CAD build for the part. Positions are in the model's coordinates, mm. Face numbers are marked on the shaded views. A direction names the side the tool comes from. Round coordinates to 2 decimals unless told otherwise and drop trailing zeros. Write each loop counter-clockwise with the first axis right and the second up, starting at its lowest first coordinate (ties: lowest second). Pieces come first, ordered by that corner, then holes. Notation, with made-up numbers: (73, -28) - (99, -28) arc R26 cw to (99, 3) - close; hole circle Ø9 at (80, 64.5). An arc over 180 degrees is marked (long way). Answer in a Markdown table with one row per item.
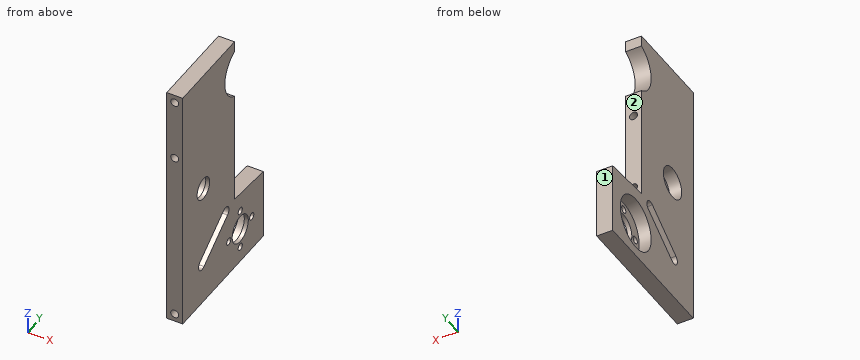
```python
from build123d import *

# Parameters (mm, degrees)
ESQUISSE2_W             = 8
ESQUISSE2_H             = 95
ESQUISSE2_H_2           = 31
BOSS_EXTRU_1_DEPTH      = 70
ESQUISSE3_R             = 7.95
ENL_V_MAT_EXTRU_1_DEPTH = 10
ESQUISSE4_R             = 13.4
ENL_V_MAT_EXTRU_2_DEPTH = 6
ESQUISSE6_R             = 1.8
ESQUISSE6_R_2           = 7
ENL_V_MAT_EXTRU_3_DEPTH = 10
ESQUISSE7_R             = 2
ENL_V_MAT_EXTRU_4_DEPTH = 15
ENL_V_MAT_EXTRU_5_DEPTH = 10
ESQUISSE9_R             = 13.4
ENL_V_MAT_EXTRU_6_DEPTH = 10
ESQUISSE10_R            = 13.4
ENL_V_MAT_EXTRU_7_DEPTH = 10
ESQUISSE12_R            = 8.1
ESQUISSE12_R_2          = 5.5
BOSS_EXTRU_3_DEPTH      = 2
ESQUISSE13_R            = 2
ENL_V_MAT_EXTRU_8_DEPTH = 15


with BuildPart() as part:
    # Esquisse2 → Boss.-Extru.1 (new body)
    with BuildSketch(Plane(origin=(0, 0, 0), x_dir=(1, 0, 0), z_dir=(0, 1, 0))):
        with Locations((4, 47.5)):
            Rectangle(ESQUISSE2_W, ESQUISSE2_H)
        with Locations((4, -15.5)):
            Rectangle(ESQUISSE2_W, ESQUISSE2_H_2)
    extrude(amount=BOSS_EXTRU_1_DEPTH)

    # Esquisse3 → Enlèv. mat.-Extru.1 (cut)
    with BuildSketch(Plane.ZY):
        with Locations((-32, 18)):
            Circle(ESQUISSE3_R)
    extrude(amount=-ENL_V_MAT_EXTRU_1_DEPTH, mode=Mode.SUBTRACT)

    # Esquisse4 → Enlèv. mat.-Extru.2 (cut)
    with BuildSketch(Plane.ZY):
        with Locations((-77, 50)):
            Circle(ESQUISSE4_R)
    extrude(amount=-ENL_V_MAT_EXTRU_2_DEPTH, mode=Mode.SUBTRACT)

    # Esquisse6 → Enlèv. mat.-Extru.3 (cut)
    with BuildSketch(Plane.ZY):
        with Locations((-77, 60)):
            Circle(ESQUISSE6_R)
        with Locations((-67, 50)):
            Circle(ESQUISSE6_R)
        with Locations((-77, 40)):
            Circle(ESQUISSE6_R)
        with Locations((-87, 50)):
            Circle(ESQUISSE6_R)
        with Locations((-77, 50)):
            Circle(ESQUISSE6_R_2)
    extrude(amount=-ENL_V_MAT_EXTRU_3_DEPTH, mode=Mode.SUBTRACT)

    # Esquisse7 → Enlèv. mat.-Extru.4 (cut)
    with BuildSketch(Plane.XZ):
        with Locations((4, -91)):
            Circle(ESQUISSE7_R)
        with Locations((4, -4)):
            Circle(ESQUISSE7_R)
        with Locations((4, 27)):
            Circle(ESQUISSE7_R)
    extrude(amount=-ENL_V_MAT_EXTRU_4_DEPTH, mode=Mode.SUBTRACT)

    # Esquisse8 → Enlèv. mat.-Extru.5 (cut)
    with BuildSketch(Plane.ZY):
        with BuildLine():
            Line((-61.528438992, 38.971206009), (-75.867849901, 18.492404902))
            ThreePointArc((-75.867849901, 18.492404902), (-75.131123077, 14.31421946), (-70.952937635, 15.050946284))
            Line((-70.952937635, 15.050946284), (-56.613526727, 35.529747391))
            ThreePointArc((-56.613526727, 35.529747391), (-57.35025355, 39.707932833), (-61.528438992, 38.971206009))
        make_face()
    extrude(amount=-ENL_V_MAT_EXTRU_5_DEPTH, mode=Mode.SUBTRACT)

    # Esquisse9 → Enlèv. mat.-Extru.6 (cut)
    with BuildSketch(Plane.ZY):
        with Locations((13, 50)):
            Circle(ESQUISSE9_R)
    extrude(amount=-ENL_V_MAT_EXTRU_6_DEPTH, mode=Mode.SUBTRACT)

    # Esquisse10 → Enlèv. mat.-Extru.7 (cut)
    with BuildSketch(Plane.ZY):
        with Locations((13, 50)):
            Circle(ESQUISSE10_R)
        Polygon((-57, 45), (-59, 70), (31, 70), (31, 45), align=None)
        with BuildLine():
            ThreePointArc((0.567783786, 45), (13, 36.6), (25.432216214, 45))
            Line((25.432216214, 45), (0.567783786, 45))
        make_face()
        with BuildLine():
            Line((0.567783786, 45), (25.432216214, 45))
            ThreePointArc((25.432216214, 45), (26.155829455, 47.453600313), (26.4, 50))
            ThreePointArc((26.4, 50), (10.453600313, 63.155829455), (0.567783786, 45))
        make_face()
    extrude(amount=-ENL_V_MAT_EXTRU_7_DEPTH, mode=Mode.SUBTRACT)

    # Esquisse12 → Boss.-Extru.3 (add)
    with BuildSketch(Plane(origin=(8, 0, 0), x_dir=(0, 0, -1), z_dir=(1, 0, 0))):
        with Locations((32, 18)):
            Circle(ESQUISSE12_R)
        with Locations((32, 18)):
            Circle(ESQUISSE12_R_2, mode=Mode.SUBTRACT)
    extrude(amount=-BOSS_EXTRU_3_DEPTH)

    # Esquisse13 → Enlèv. mat.-Extru.8 (cut)
    with BuildSketch(Plane(origin=(0, 45, 0), x_dir=(1, 0, 0), z_dir=(0, 1, 0))):
        with Locations((4, 12)):
            Circle(ESQUISSE13_R)
        with Locations((4, 52)):
            Circle(ESQUISSE13_R)
    extrude(amount=-ENL_V_MAT_EXTRU_8_DEPTH, mode=Mode.SUBTRACT)


solid = part.part
```
Q1. Drill centre lines: line 1 (Y direction, x = 6.65, z = -77); line 2 (Z direction, x = 4, y = 4); line 3 (Y direction, x = 4.25, z = -68.5). Where is each one in solid material? Low to high.
Computed:
| item | result |
|---|---|
| line 1 | y = 0 to 38.2, 41.8 to 43, 57 to 58.2, 61.8 to 70 |
| line 2 | z = -95 to -93, -89 to -6, -2 to 25, 29 to 31 |
| line 3 | y = 0 to 18.55, 29.01 to 39.64, 60.36 to 70 |
Q2. Saw through at C-C on y = 6. List the corners of the cut face in (x, z).
Computed:
| item | result |
|---|---|
| outline | (0, -95) - (8, -95) - (8, 31) - (0, 31) - close; hole circle Ø4 at (4, -91); hole circle Ø4 at (4, -4); hole circle Ø4 at (4, 27) |
Q3. Saw through at B-B on y = 31.5. List the corners of the cut face in (x, z), then the cut area to 3 significant figures.
Computed:
| item | result |
|---|---|
| outline | (0, -95) - (8, -95) - (8, -66.76) - (0, -66.76) - close; (0, -59.44) - (8, -59.44) - (8, 31) - (0, 31) - close; hole circle Ø4 at (4, -52); hole circle Ø4 at (4, -12) |
| area | 924 mm2 |
Q4. 3-axis set-ups, long thin cutter, end or side, ignore diameter. For the marked faces 1 and 2: which of +Z, -Z, +X, -X, +Y, -Y reach the whole face in a straight line?
Computed:
| item | result |
|---|---|
| face 1 | +Z, -Z, +X, -X, +Y |
| face 2 | +Z, +X, -X, +Y |
Q5. Saw through at A-A on x = 4. Count the separate pieces of the cut face and the enclosed holes in it, then the cut area to 3 significant figures.
Computed:
| item | result |
|---|---|
| separate pieces | 1 |
| enclosed holes | 3 |
| area | 5,200 mm2 |
Q6. Flat gauge pins, fed straight in: pin 1 (4 mm diameter, centred on x = 4.5, z = -27, fed in from +Y); pin 2 (4 mm diameter, centred on y = 50, z = -87, fed in from -X). Where does each tip first touch, or does it go through?
Computed:
| item | result |
|---|---|
| pin 1 | stops at y = 45 |
| pin 2 | stops at x = 6 |
Q7. Saw through at D-D on z = 27. List the corners of the cut face in (x, y).
Computed:
| item | result |
|---|---|
| outline | (0, 0) - (2, 0) - (2, 15) - (6, 15) - (6, 0) - (8, 0) - (8, 45) - (0, 45) - close |
